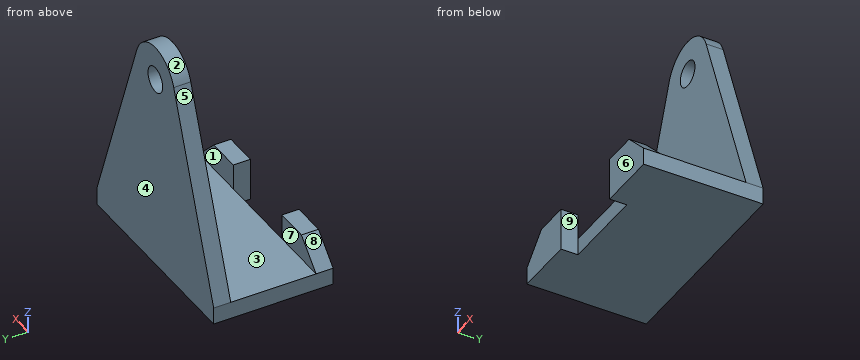
```python
from build123d import *

# Parameters (mm, degrees)
F0_R     = 7.5
F0_W     = 120
F0_H     = 10
F1_DEPTH = 10
F2_W     = 120
F2_H     = 10
F3_DEPTH = 50
F4_W     = 35
F4_H     = 10
F5_DEPTH = 10


with BuildPart() as f1:
    # F0 (on Front) → F1 (new body)
    with BuildSketch(Plane.XZ):
        with BuildLine():
            Line((-20.090676, 74.255499), (-61.133094, -38.507616))
            Line((-61.133094, -38.507616), (58.866906, -38.507616))
            Line((58.866906, -38.507616), (17.824489, 74.255499))
            ThreePointArc((17.824489, 74.255499), (-1.133094, 87.529741), (-20.090676, 74.255499))
        make_face()
        with Locations((-1.133094, 67.355503)):
            Circle(F0_R, mode=Mode.SUBTRACT)
        with Locations((-1.133094, -43.507616)):
            Rectangle(F0_W, F0_H)
    extrude(amount=F1_DEPTH)

    # F2 (on face) → F3 (join)
    with BuildSketch(Plane.XZ.offset(10)):
        with Locations((-1.133094, -43.507616)):
            Rectangle(F2_W, F2_H)
    extrude(amount=F3_DEPTH)

    # F4 (on face) → F5 (join)
    with BuildSketch(Plane.XZ.offset(60)):
        Polygon((23.866906, -23.507616), (23.866906, -38.507616), (58.866906, -38.507616), (43.866906, -23.507616), align=None)
        with Locations((-43.633094, -43.507616)):
            Rectangle(F4_W, F4_H)
        with Locations((41.366906, -43.507616)):
            Rectangle(F4_W, F4_H)
        Polygon((-46.133094, -23.507616), (-61.133094, -38.507616), (-26.133094, -38.507616), (-26.133094, -23.507616), align=None)
    extrude(amount=F5_DEPTH)


solid = f1.part
```
Model file for the job. Use its own axes, mm. Face numbers are marked on the shaded views. A direction names the side the tool comes from. Give positions to 0.01 mm unless a question says otherwise; leave off trailing zeros. Write each loop counter-clockwise with the first axis right and the second up, starting at its lowest first coordinate (ties: lowest second). Pieces come first, ordered by that corner, then holes. Notation, with made-up numbers: M 30,15 L 78,15 A13 ccw 78,22 Z; hole C 72.25,12 d10. An arc over 180 degrees is marked long. Use a Markdown table: item, result.
1) Cut at B-B (x = -3). List the corners of the cut face in (y, z), and give its area (3 significant figures).
Responses:
| item | result |
|---|---|
| outline | M -60,-48.51 L 0,-48.51 L 0,60.09 L -10,60.09 L -10,-38.51 L -60,-38.51 Z; M -10,74.62 L 0,74.62 L 0,87.44 L -10,87.44 Z |
| area | 1,710 mm2 |
2) Drill centre lines: line 1 (Y direction, x = 12.5, z = 20); line 2 (Z direction, x = -11, y = -58); line 3 (Z direction, x = -30.5, y = -66). Where is each one in solid material? Low to high. Write a range as from..to.
Responses:
| item | result |
|---|---|
| line 1 | y = -10..0 |
| line 2 | z = -48.51..-38.51 |
| line 3 | z = -48.51..-23.51 |
3) Pull direction Y, two halves, no side cores. Call the marked faces 1, 2, 3 and 4: +Y half, -Y half, draft (parallel to the pull), parting line (faces both ways), or undercut.
Responses:
| item | result |
|---|---|
| face 1 | undercut |
| face 2 | draft |
| face 3 | undercut |
| face 4 | +Y half |
4) Cut at D-D (y = -51.5). List the corners of the cut face in (x, z), and give its area (3 significant figures).
Responses:
| item | result |
|---|---|
| outline | M -61.13,-48.51 L 58.87,-48.51 L 58.87,-38.51 L -61.13,-38.51 Z |
| area | 1,200 mm2 |
5) Cut at A-A (y = -62). List the corners of the cut face in (x, z).
Responses:
| item | result |
|---|---|
| outline | M -61.13,-48.51 L -26.13,-48.51 L -26.13,-23.51 L -46.13,-23.51 L -61.13,-38.51 Z; M 23.87,-48.51 L 58.87,-48.51 L 58.87,-38.51 L 43.87,-23.51 L 23.87,-23.51 Z |
6) Tool access for the marked faces 5, 6, 7, 8 and 9: list every direction of +Z, -Z, +X, -X, +Y, -Y with a clear straight run to the whole face (end or side of a thin tool).
Responses:
| item | result |
|---|---|
| face 5 | +Z, -X, +Y, -Y |
| face 6 | +Z, -Z, +X, -X, -Y |
| face 7 | +Z, +X, -X |
| face 8 | +Z, -X, -Y |
| face 9 | +Z, -Z, -Y |
7) Pin check, flat tips, straight feed: pin 1 (8 mm diameter, centred on x = -2, z = -45.5, fed in from -Y); pin 2 (5 mm diameter, centred on y = -65, z = -37, fed in from +X); pin 3 (9 mm diameter, centred on x = -1.13, z = 67.36, fed in from -Y); pin 4 (1 mm diameter, centred on x = -0.5, z = 30, fed in from -Y). Stop position of each tip, or through.
Responses:
| item | result |
|---|---|
| pin 1 | stops at y = -60 |
| pin 2 | stops at x = 58.87 |
| pin 3 | passes through |
| pin 4 | stops at y = -10 |
8) Cut at C-C (x = 28). List the corners of the cut face in (y, z).
Responses:
| item | result |
|---|---|
| outline | M -70,-48.51 L 0,-48.51 L 0,46.3 L -10,46.3 L -10,-38.51 L -60,-38.51 L -60,-23.51 L -70,-23.51 Z |
